from build123d import *

# Parameters (mm, degrees)
SKETCH1_R                = 38.1
HUB_CENTER_DEPTH         = 25.4
HUB_CENTER_DEPTH_BACK    = 23.4
INNER_START              = 1.397
SKETCH2_R                = 46.99
INNER_BEARING_DEPTH      = 13.208
OUTER_START              = -1.397
SKETCH3_R                = 46.99
OUTER_BEARING_DEPTH      = 13.208
TIRE_ARM_DEPTH           = 2.54
SKETCH5_W                = 25.4
SKETCH5_H                = 203.2
TIRE_CONTACT_PATCH_DEPTH = 2.54


with BuildPart() as part:
    # Sketch1 → Hub Center (new body, two sides)
    with BuildSketch(Plane.XY) as hub_center_sk:
        Circle(SKETCH1_R)
    extrude(amount=HUB_CENTER_DEPTH)
    extrude(hub_center_sk.sketch, amount=-HUB_CENTER_DEPTH_BACK)

    # Sketch2 → Inner Bearing (add)
    with BuildSketch(Plane.XY.offset(INNER_START)):
        Circle(SKETCH2_R)
    extrude(amount=INNER_BEARING_DEPTH)

    # Sketch3 → Outer Bearing (add)
    with BuildSketch(Plane.XY.offset(OUTER_START)):
        Circle(SKETCH3_R)
    extrude(amount=-OUTER_BEARING_DEPTH)

    # Sketch4 → Tire Arm (add)
    with BuildSketch(Plane(origin=(0, 0, -23.4), x_dir=(-1, 0, 0), z_dir=(0, 0, -1))):
        with BuildLine():
            Line((-12.7, -35.921024484), (-12.7, -261.62))
            Line((-12.7, -261.62), (12.7, -261.62))
            Line((12.7, -261.62), (12.7, -35.921024484))
            ThreePointArc((12.7, -35.921024484), (0, -38.1), (-12.7, -35.921024484))
        make_face()
    extrude(amount=-TIRE_ARM_DEPTH)

    # Sketch5 → Tire Contact Patch (add)
    with BuildSketch(Plane.XZ.offset(261.62)):
        with Locations((0, -22.13)):
            Rectangle(SKETCH5_W, SKETCH5_H)
    extrude(amount=-TIRE_CONTACT_PATCH_DEPTH)


solid = part.part
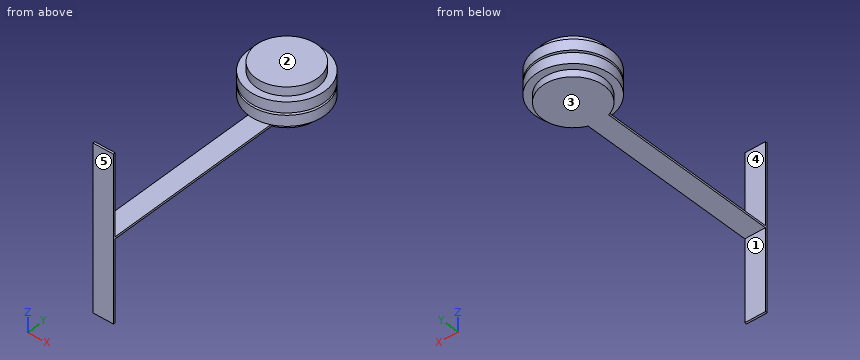
Could you check a few things on this model? Use its own coordinates, in mm. Face numbers are marked on the shaded views. A direction names the side the tool comes from. Give positions to 0.01 mm unless a question says otherwise; leave off trailing zeros. Order: outer loops, then holes, each group sorted by start corner. A loop starts at its lowest first (then second) coordinate and runs counter-clockwise, first axis right, second up.
Item 1: I need wall thicknesses on line 1 (Y direction, x = -8, z = -37.5); line 2 (Z direction, x = -5, y = -172); line 3 (X direction, y = -2.5, z = -4.5). Which ranges of each line are inside material? Lowest first, please.
Item 2: If we section it at A-A, the plane x = 0: Write out the boundary of the cut face in (y, z) (3 decimals), plus the area to 3 significant figures.
Item 3: For the marked faces 1 and 2, which set-ups out of +Z, -Z, +X, -X, +Y, -Y let a thin tool reach every point of the face, with its end or its side?
Item 4: If we section it at C-C, the plane z = -105: Write out the boundary of the cut face in (x, y), plus the area to 3 significant figures.
Item 5: If we section it at B-B, the plane y = 0: Write out the boundary of the cut face in (x, z) (3 decimals), plus the area to 3 significant figures.
Item 6: If we section it at D-D, the plane x = -34.5: Write out the boundary of the cut face in (y, z) (3 decimals), plus the area to 3 significant figures.
Item 7: If we mould it in two halves opening along Y, with no side actions, what happens to the marked faces 3, 4 and 5? For each: pulls with the +Y half, pulls with the -Y half, needs draft (parallel to the pull), parting line crosses it, or undercut.
Item 8: I'm going to push flat-ended pins straight in: pin 1 (1.5 mm diameter, centred on y = -171.5, z = -18.5, fed in from +X); pin 2 (20.5 mm diameter, centred on x = -6, z = -59.5, fed in from +Y); pin 3 (3 mm diameter, centred on x = -26.5, z = -8, fed in from -Y); pin 4 (1 mm diameter, centred on x = -3.5, y = -148, fed in from +Z). Where does each tip first touch, or does it pass through?
Values:
1. line 1: y = -261.62 to -259.08
1. line 2: z = -23.4 to -20.86
1. line 3: x = -46.92 to 46.92
2. outline: (-261.62, -123.73) - (-259.08, -123.73) - (-259.08, -23.4) - (38.1, -23.4) - (38.1, -14.605) - (46.99, -14.605) - (46.99, -1.397) - (38.1, -1.397) - (38.1, 1.397) - (46.99, 1.397) - (46.99, 14.605) - (38.1, 14.605) - (38.1, 25.4) - (-38.1, 25.4) - (-38.1, 14.605) - (-46.99, 14.605) - (-46.99, 1.397) - (-38.1, 1.397) - (-38.1, -1.397) - (-46.99, -1.397) - (-46.99, -14.605) - (-38.1, -14.605) - (-38.1, -20.86) - (-259.08, -20.86) - (-259.08, 79.47) - (-261.62, 79.47) - close
2. area: 5,270 mm2
3. face 1: -Z, +X, -X, +Y
3. face 2: +Z, +X, -X, +Y
4. outline: (-12.7, -261.62) - (12.7, -261.62) - (12.7, -259.08) - (-12.7, -259.08) - close
4. area: 64.5 mm2
5. outline: (-46.99, -14.605) - (-38.1, -14.605) - (-38.1, -23.4) - (38.1, -23.4) - (38.1, -14.605) - (46.99, -14.605) - (46.99, -1.397) - (38.1, -1.397) - (38.1, 1.397) - (46.99, 1.397) - (46.99, 14.605) - (38.1, 14.605) - (38.1, 25.4) - (-38.1, 25.4) - (-38.1, 14.605) - (-46.99, 14.605) - (-46.99, 1.397) - (-38.1, 1.397) - (-38.1, -1.397) - (-46.99, -1.397) - close
5. area: 4,190 mm2
6. outline: (-31.903, -14.605) - (-16.167, -14.605) - (-16.167, -23.4) - (16.167, -23.4) - (16.167, -14.605) - (31.903, -14.605) - (31.903, -1.397) - (16.167, -1.397) - (16.167, 1.397) - (31.903, 1.397) - (31.903, 14.605) - (16.167, 14.605) - (16.167, 25.4) - (-16.167, 25.4) - (-16.167, 14.605) - (-31.903, 14.605) - (-31.903, 1.397) - (-16.167, 1.397) - (-16.167, -1.397) - (-31.903, -1.397) - close
6. area: 2,410 mm2
7. face 3: needs draft
7. face 4: undercut
7. face 5: pulls with the -Y half
8. pin 1: passes through
8. pin 2: stops at y = -259.08
8. pin 3: stops at y = -39.79
8. pin 4: stops at z = -20.86
